The drawing under review shows one solid part. Ordinate dimensions are in mm from its lowest x, y, z. A direction names the side the tool comes from. Coordinates: 2 decimals unless noted, no trailing zeros. Write each loop counter-clockwise with the first axis right and the second up, starting at its lowest first coordinate (ties: lowest second). Pieces come first, ordered by that corner, then holes.
Q1. For probe 1 along X at (y, z) = (49.5, 4); probe 2 along X at (y, z) = (50.5, 41); probe 3 along Z at (x, y) = (60, 143), list the stretches that pass through material, from the lowest coordinate up.
Q2. Take a section at C-C (y = 47). Give the boundary of the cut face in (x, z).
Q3. Machinability: for the marked faces 1, 2, 3 and 4, which of the approach directions +Z, -Z, +X, -X, +Y, -Y give a long, thin tool a straight path to every point of the face, cutting with its end or side? Answer none if there is none.
Q4. Take a section at A-A (z = 16). Give the boundary of the cut face in (x, y).
Q5. Take a section at B-B (x = 108.5). Give the boundary of the cut face in (y, z), and give its area (3 significant figures).
Q6. Take a section at D-D (x = 190). Give the boundary of the cut face in (y, z).
Q7. Insertion check: pin 1 (10 mm diameter, centred on x = 123.5, y = 209, fed in from +Z); pin 2 (6 mm diameter, centred on y = 222, z = 9, fed in from +X); pin 3 (16 mm diameter, centred on y = 203.5, z = 9.5, fed in from -X). Each pin has a flat end and moves straight along its axis. Give the tip position at first contact, or say it passes through.
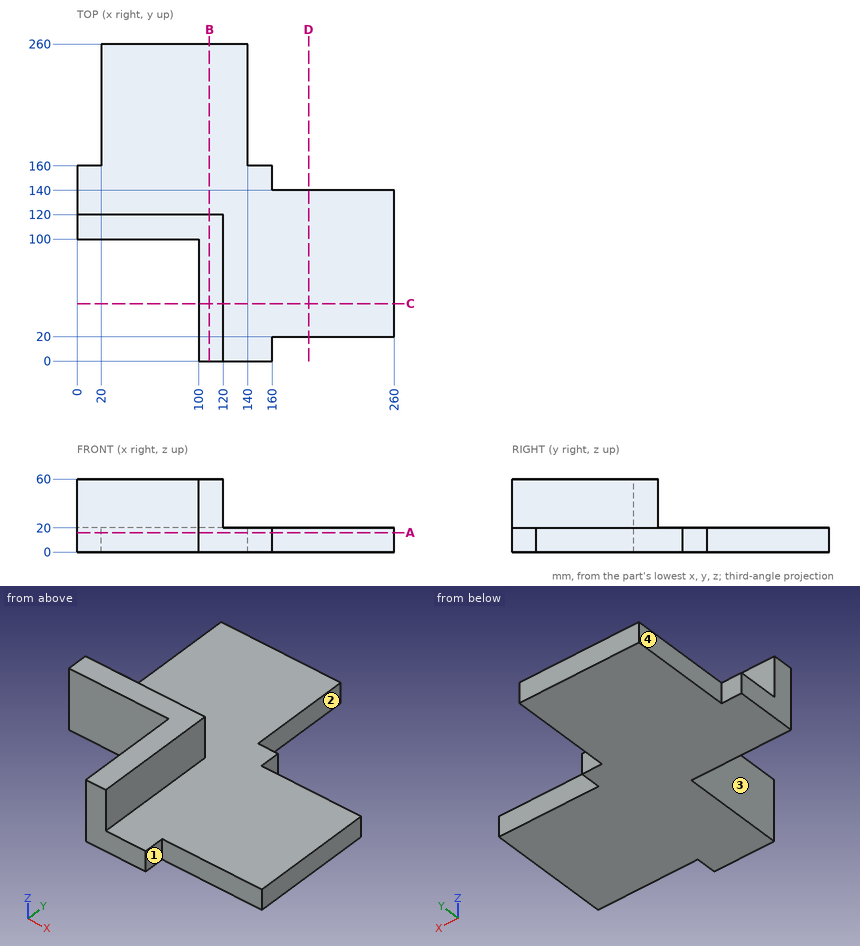
Response:
1. probe 1: x = 100 to 260
1. probe 2: x = 100 to 120
1. probe 3: z = 0 to 20
2. outline: (100, 0) - (260, 0) - (260, 20) - (120, 20) - (120, 60) - (100, 60) - close
3. face 1: +Z, -Z, +X, -Y
3. face 2: +Z, -Z, +X, +Y
3. face 3: +Z, -Z, -X, -Y
3. face 4: +Z, -Z, -X, +Y
4. outline: (0, 100) - (100, 100) - (100, 0) - (160, 0) - (160, 20) - (260, 20) - (260, 140) - (160, 140) - (160, 160) - (140, 160) - (140, 260) - (20, 260) - (20, 160) - (0, 160) - close
5. outline: (0, 0) - (260, 0) - (260, 20) - (120, 20) - (120, 60) - (0, 60) - close
5. area: 10,000 mm2
6. outline: (20, 0) - (140, 0) - (140, 20) - (20, 20) - close
7. pin 1: stops at z = 20
7. pin 2: stops at x = 140
7. pin 3: stops at x = 20
